Autodesk Inventor part; units mm, degrees
ref_plane "YZ Plane" through (0, 0, 0) normal (1, 0, 0) x (0, 1, 0)
ref_plane "XZ Plane" through (0, 0, 0) normal (0, 1, 0) x (-1, 0, 0)
ref_plane "XY Plane" through (0, 0, 0) normal (0, 0, 1) x (1, 0, 0)
sketch "スケッチ1" plane through (0, 0, 0) normal (0, 1, 0) x (-1, 0, 0)
  arc A0 (182.3045, -62.8657) -> (348.4892, -47.2216) centre (162.2533, 1040.6287) ccw
  arc A1 (135.2834, -62.3282) -> (182.3045, -62.8657) centre (167.871, 731.467) ccw
  arc A2 (49.3906, -47.0603) -> (135.2834, -62.3282) centre (148.588, 261.756) ccw
  arc A3 (0.1309, -22.8654) -> (49.3906, -47.0603) centre (107.173, 132.825) ccw
  arc A4 (-13.3538, -9.7713) -> (0.1309, -22.8654) centre (31.9, 23.342) ccw
  arc A5 (-7.3318, 8.7424) -> (-13.3538, -9.7713) centre (-3.6695, -2.6851) ccw
  arc A6 (12.9042, 11.391) -> (-7.3318, 8.7424) centre (10.0641, -45.5382) ccw
  arc A7 (90.1175, -2.8524) -> (12.9042, 11.391) centre (-1.8944, -285.2401) ccw
  arc A8 (90.1175, -2.8524) -> (94.8834, -4.3943) centre (462.8125, 1140.9603) ccw
  arc A9 (94.8834, -4.3943) -> (348.3291, -45.236) centre (355.7675, 807.7316) ccw
  arc A10 (348.4892, -47.2216) -> (348.3291, -45.236) centre (348.3204, -46.2359) ccw
  circle A11 centre (29.3651, -6.1392) radius 6
  circle A12 centre (239.8151, -50.1371) radius 6
  point P0 (0, 0)
extrude "押し出し1" add sketch "スケッチ1" along normal mid plane 41.5
properties part number "uretan_m" material "ポリエチレン、高密度"
Input: part model. Units: mm. Frame: model coordinates. Coordinates: 2 decimals unless noted, no trailing zeros. Write each loop counter-clockwise with the first axis right and the second up, starting at its lowest first coordinate (ties: lowest second). Pieces come first, ordered by that corner, then holes. Notation, with made-up numbers: (64, 78) - (96, 78) arc R24 cw to (96, 98) - close; hole circle Ø4 at (56, -3.5). An arc over 180 degrees is marked (long way). Put each result on its own line as item: value. Start each with the question number.
1) Contact query for flat-ended pins moving along their axis: pin 1 (1.5 mm diameter, centred on x = -218.5, y = -13.5, fed in from +Z); pin 2 (5 mm diameter, centred on y = 11, z = -34.5, fed in from +X); pin 3 (7 mm diameter, centred on x = -239.82, z = -50.14, fed in from -Y); pin 4 (1 mm diameter, centred on x = -124, y = -10.5, fed in from +Z). Output: stop coordinate, or through.
2) Cut plane C-C (z = -18.5). Return the cut outline in (x, y).
3) Cut plane B-B (x = -32). Return the cut outline in (y, z).
4) Cut plane D-D (x = -160). Return the cut outline in (y, z), plus the area to 3 significant figures.
5) Ray query, L1, parallel to Z at x = -145, y = 2; L2, parallel to Z at x = -7, y = 14. Return the intervals inside material, ascending.
6) Cut plane A-A (y = -6). Return the cut outline in (x, z).
7) Mould query, pull axis Z, two halves, no side actions, for faces 1 (the face through (-221.84, -0.29, -34.69)), 2 (the face through (-23.37, -0.29, -6.4)), 3 (the face through (15.129, -0.291, 0.875)), 4 (the face through (-92.42, -0.29, -57.7)). Classes: pulls with the +Z half, pulls with the -Z half, needs draft (parallel to the pull), parting line crosses it, or undercut.
Resolved:
1. pin 1: stops at z = -34.03
1. pin 2: stops at x = -14.81
1. pin 3: passes through
1. pin 4: stops at z = -13.04
2. outline: (-143.75, -20.75) - (5.43, -20.75) - (5.43, 20.75) - (-143.75, 20.75) - close
3. outline: (-20.75, -40.51) - (20.75, -40.51) - (20.75, -11.53) - (-20.75, -11.53) - close; (-20.75, -0.75) - (20.75, -0.75) - (20.75, 9.82) - (-20.75, 9.82) - close
4. outline: (-20.75, -62.96) - (20.75, -62.96) - (20.75, -22.5) - (-20.75, -22.5) - close
4. area: 1,680 mm2
5. L1: z = -62.67 to -18.82
5. L2: z = -27.37 to 11.38
6. outline: (-348.49, -47.22) arc R1103.69 ccw to (-182.3, -62.87) arc R794.46 ccw to (-135.28, -62.33) arc R324.35 ccw to (-49.39, -47.06) arc R188.94 ccw to (-0.13, -22.87) arc R56.08 ccw to (13.35, -9.77) arc R12 ccw to (7.33, 8.74) arc R57 ccw to (-12.9, 11.39) arc R297 ccw to (-90.12, -2.85) arc R1196.01 cw to (-94.88, -4.39) arc R853 cw to (-348.33, -45.24) arc R1 ccw to start; hole circle Ø12 at (-239.82, -50.14); hole circle Ø12 at (-29.37, -6.14)
7. face 1: pulls with the +Z half
7. face 2: undercut
7. face 3: parting line crosses it
7. face 4: pulls with the -Z half
